Here's how the part is built. I have some questions about the finished solid (model axes, mm). Face numbers are marked on the shaded views. Give positions to 0.01 mm unless a question says otherwise; leave off trailing zeros. Write each loop counter-clockwise with the first axis right and the second up, starting at its lowest first coordinate (ties: lowest second). Pieces come first, ordered by that corner, then holes. Notation, with made-up numbers: (29, 64) - (77, 64) arc R31 ccw to (77, 95) - close; hole circle Ø6 at (67.25, 51). An arc over 180 degrees is marked (long way). Use a Markdown table: item, result.
```python
from build123d import *

# Parameters (mm, degrees)
BOSS_EXTRUDE1_START = -2.2225
SKETCH2_R           = 3.175
SKETCH2_R_2         = 1.2446
BOSS_EXTRUDE1_DEPTH = 2.2225
SKETCH3_R           = 2.731389
SKETCH3_R_2         = 1.2446
BOSS_EXTRUDE2_DEPTH = 0.635
FILLET1_R           = 0.381
FILLET2_R           = 0.381
CHAMFER1_SIZE       = 0.381


with BuildPart() as part:
    # Sketch1 → Revolve1 (revolve)
    with BuildSketch(Plane.XY, mode=Mode.PRIVATE) as revolve1_sk:
        with BuildLine():
            Line((0, 2.731389), (0, 1.2446))
            Line((0, 1.2446), (-5.7531, 1.2446))
            Line((-5.7531, 1.2446), (-5.7531, 3.175))
            Line((-5.7531, 3.175), (-3.5306, 3.175))
            Line((-3.5306, 3.175), (-3.5306, 2.731389))
            ThreePointArc((-3.5306, 2.731389), (-1.7653, 3.047974688), (0, 2.731389))
        make_face()
    revolve(revolve1_sk.sketch.rotate(Axis((-40.930080617, 0, 0), (1, 0, 0)), 90), axis=Axis((-40.930080617, 0, 0), (1, 0, 0)))

    # Sketch2 → Boss-Extrude1 (add)
    # profile 1 of 7: a face of its own
    with BuildSketch(Plane.ZY.offset(5.7531).offset(BOSS_EXTRUDE1_START)):
        with BuildLine():
            Line((1.587499954, 2.749630684), (0, 3.666174209))
            Line((0, 3.666174209), (-1.587500022, 2.749630644))
            ThreePointArc((-1.587500022, 2.749630644), (-3.9e-08, 3.175), (1.587499954, 2.749630684))
        make_face()
    # profile 2 of 7: a face of its own
    with BuildSketch(Plane.ZY.offset(5.7531).offset(BOSS_EXTRUDE1_START)):
        with BuildLine():
            ThreePointArc((-3.175, 0), (-2.749630663, 1.587499989), (-1.587500022, 2.749630644))
            Line((-1.587500022, 2.749630644), (-3.175, 1.833087105))
            Line((-3.175, 1.833087105), (-3.175, 0))
        make_face()
    # profile 3 of 7: a face of its own
    with BuildSketch(Plane.ZY.offset(5.7531).offset(BOSS_EXTRUDE1_START)):
        with BuildLine():
            ThreePointArc((-1.587499933, -2.749630696), (-2.749630638, -1.587500034), (-3.175, 0))
            Line((-3.175, 0), (-3.175, -1.833087105))
            Line((-3.175, -1.833087105), (-1.587499933, -2.749630696))
        make_face()
    # profile 4 of 7: a face of its own
    with BuildSketch(Plane.ZY.offset(5.7531).offset(BOSS_EXTRUDE1_START)):
        with BuildLine():
            ThreePointArc((1.587499954, -2.749630684), (1.2e-08, -3.175), (-1.587499933, -2.749630696))
            Line((-1.587499933, -2.749630696), (0, -3.666174209))
            Line((0, -3.666174209), (1.587499954, -2.749630684))
        make_face()
    # profile 5 of 7: a face of its own
    with BuildSketch(Plane.ZY.offset(5.7531).offset(BOSS_EXTRUDE1_START)):
        with BuildLine():
            Line((3.175, -1.833087105), (3.175, 0))
            ThreePointArc((3.175, 0), (2.749630644, -1.587500023), (1.587499954, -2.749630684))
            Line((1.587499954, -2.749630684), (3.175, -1.833087105))
        make_face()
    # profile 6 of 7: a face of its own
    with BuildSketch(Plane.ZY.offset(5.7531).offset(BOSS_EXTRUDE1_START)):
        with BuildLine():
            Line((3.175, 1.833087105), (1.587499954, 2.749630684))
            ThreePointArc((1.587499954, 2.749630684), (2.749630644, 1.587500023), (3.175, 0))
            Line((3.175, 0), (3.175, 1.833087105))
        make_face()
    # profile 7 of 7: a face of its own
    with BuildSketch(Plane.ZY.offset(5.7531).offset(BOSS_EXTRUDE1_START)):
        Circle(SKETCH2_R)
        Circle(SKETCH2_R_2, mode=Mode.SUBTRACT)
    extrude(amount=BOSS_EXTRUDE1_DEPTH)

    # Sketch3 → Boss-Extrude2 (add)
    with BuildSketch(Plane(origin=(0, 0, 0), x_dir=(0, 0, -1), z_dir=(1, 0, 0))):
        Circle(SKETCH3_R)
        with Locations(Location((0, 0, 0), (0, 0, 180))):
            Circle(SKETCH3_R_2, mode=Mode.SUBTRACT)
    extrude(amount=BOSS_EXTRUDE2_DEPTH)

    # Fillet1
    # the kernel refuses this fillet: 0.381 mm, written as the material it adds along each edge
    with BuildSketch(Plane(origin=(-3.5306, 0, 0), x_dir=(0, 0, 1), z_dir=(0, 1, 0))) as fillet1_piece_1_section:
        with BuildLine():
            CenterArc((3.250609874, 0.381), FILLET1_R, 165.315967452, 104.684032548)
            Line((3.250609874, 0), (2.731389, 0))
            ThreePointArc((2.731389, 0), (2.81260995, 0.236931857), (2.882053931, 0.47757907))
        make_face()
    fillet1_piece_1 = revolve(axis=Axis((-3.5306, 0, 0), (1, 0, 0)), mode=Mode.PRIVATE)
    fillet1_piece_1 = split(fillet1_piece_1, bisect_by=Plane(origin=(-3.388898911, -4.022914712, -0.617892675), z_dir=(0, 0.8660254037844387, -0.49999999999999994)), keep=Keep.TOP, mode=Mode.PRIVATE)
    fillet1_piece_1 = split(fillet1_piece_1, bisect_by=Plane(origin=(-3.388898911, -1.476346602, -3.792892675), z_dir=(0, 0.8660254037844389, 0.4999999999999997)), keep=Keep.TOP, mode=Mode.PRIVATE)
    fillet1_piece_1 = split(fillet1_piece_1, bisect_by=Plane(origin=(-3.388898911, 0, -3.175), z_dir=(0, 0, 1)), keep=Keep.TOP, mode=Mode.PRIVATE)
    fillet1_piece_1 = split(fillet1_piece_1, bisect_by=Plane(origin=(-3.388898911, 1.476346602, -3.792892675), z_dir=(0, -0.8660254037844386, 0.5000000000000001)), keep=Keep.TOP, mode=Mode.PRIVATE)
    fillet1_piece_1 = split(fillet1_piece_1, bisect_by=Plane(origin=(-3.388898911, 4.022914712, -0.617892675), z_dir=(0, -0.8660254037844387, -0.49999999999999983)), keep=Keep.TOP, mode=Mode.PRIVATE)
    fillet1_piece_1 = split(fillet1_piece_1, bisect_by=Plane(origin=(-3.388898911, 0, 3.175), z_dir=(0, 0, -1)), keep=Keep.TOP, mode=Mode.PRIVATE)
    add(fillet1_piece_1)

    # Fillet2
    fillet2_edges = [part.edges().sort_by_distance(p)[0] for p in [
        (0, -2.731389, 0),
    ]]
    fillet(fillet2_edges, radius=FILLET2_R)

    # Chamfer1
    chamfer1_edges = [part.edges().sort_by_distance(p)[0] for p in [
        (0.635, 0, -1.2446),
    ]]
    chamfer(chamfer1_edges, length=CHAMFER1_SIZE)


solid = part.part
```
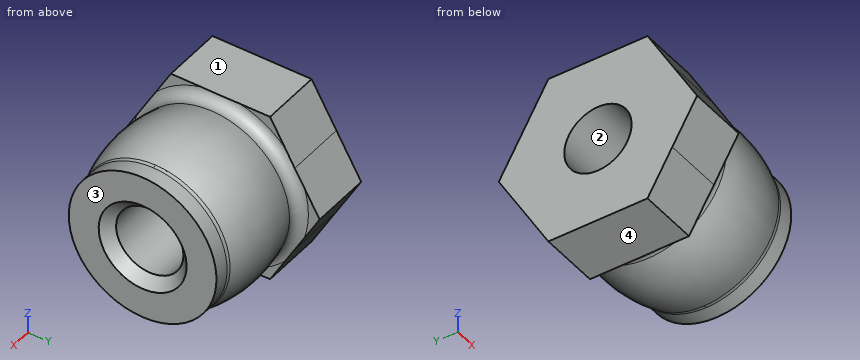
Item 1: Thinking about a two-plate mould opening in Z: for the marked faces 1, 2, 3 and 4, which applies, +Z half, -Z half, draft (parallel to the pull), parting line (faces both ways), or undercut?
Values:
| item | result |
|---|---|
| face 1 | +Z half |
| face 2 | undercut |
| face 3 | draft |
| face 4 | -Z half |
Item 2: If we section it at A-A, the plane x = -4.75: Write out the boundary of the cut face in (y, z) (1 decimal), plus the area to 3 significant figures.
Values:
| item | result |
|---|---|
| outline | (-3.7, 0) - (-1.8, -3.2) - (1.8, -3.2) - (3.7, 0) - (1.8, 3.2) - (-1.8, 3.2) - close; hole circle Ø2.5 at (0, 0) |
| area | 30.1 mm2 |
Item 3: Will these pins go through, and if not, where does the flat tip stop? pin 1 Ø0.6 at (y, z) = (-3.5, -0.5) entering from +X; pin 2 Ø1 at (x, y) = (-1, -1) entering from +Z.
Values:
| item | result |
|---|---|
| pin 1 | stops at x = -3.53 |
| pin 2 | stops at z = 2.97 |
Item 4: I need wall thicknesses on line 1 along Y through (x, z) = (-1, -0.5); line 2 along Y through (x, z) = (-5, -1); line 3 along Y through (x, z) = (-5.5, 1.5). Which ranges of each line are inside material? Lowest first, please. Write a range as [from, to].
Values:
| item | result |
|---|---|
| line 1 | y = [-2.95, -1.14], [1.14, 2.95] |
| line 2 | y = [-3.09, -0.74], [0.74, 3.09] |
| line 3 | y = [-2.8, 2.8] |
